Here's how the part is built. I have some questions about the finished solid (model axes, mm). Give positions to 0.01 mm unless a question says otherwise; leave off trailing zeros. Write each loop counter-clockwise with the first axis right and the second up, starting at its lowest first coordinate (ties: lowest second). Pieces come first, ordered by that corner, then holes. Notation, with made-up numbers: (-11, -6.75) - (11, -6.75) arc R26 cw to (11, 15.25) - close; hole circle Ø6 at (-28, 29.5). An arc over 180 degrees is marked (long way). One line per item, written item: value. Start each with the question number.
1) Imagine slicing it at D-D on y = 3.95. Write out the boundary of the cut face in (x, z).
2) Imagine slicing it at B-B on z = -89.34. Write out the boundary of the cut face in (x, y).
3) Please list where these lines run through material, in increasing order: L1, parallel to X at y = 1.5, z = -63; L2, parallel to X at y = 3.5, z = -129.34; L3, parallel to X at y = 1.45, z = -105. Write a range as [from, to].
4) Imagine slicing it at A-A on x = -180. Write out the boundary of the cut face in (y, z), plus the area to 3 significant figures.
5) I'm going to push a flat-ended pin straight in: P1, Ø1.8, axis at y = 2, z = -95, coming from the +X side. Where does the tip first touch, or does it pass through?
6) Imagine slicing it at C-C on z = -65. Write out the boundary of the cut face in (x, y), plus the area to 3 significant figures.
Autodesk Inventor part; units mm, degrees
ref_plane "YZ Plane" through (0, 0, 0) normal (1, 0, 0) x (0, 1, 0)
ref_plane "XZ Plane" through (0, 0, 0) normal (0, 1, 0) x (-1, 0, 0)
ref_plane "XY Plane" through (0, 0, 0) normal (0, 0, 1) x (1, 0, 0)
sketch "Sketch1" plane through (0, 0, 0) normal (0, 1, 0) x (-1, 0, 0)
  line L0 (232.1908, -176.5808) -> (232.1908, -3.7592)
  arc A0 (232.1908, -3.7592) -> (227.4316, 1) centre (227.4316, -3.7592) ccw
  line L1 (227.4316, 1) -> (0, 1)
  arc A1 (0, 1) -> (-4.7592, -3.7592) centre (0, -3.7592) ccw
  arc A2 (-4.7592, -176.5808) -> (0, -181.34) centre (0, -176.5808) ccw
  arc A3 (227.4316, -181.34) -> (232.1908, -176.5808) centre (227.4316, -176.5808) ccw
  circle A4 centre (130, -129.34) radius 2.25
  circle A5 centre (130, -89.34) radius 2.25
  circle A6 centre (90, -129.34) radius 2.25
  circle A7 centre (90, -89.34) radius 2.25
  circle A8 centre (180, -110) radius 3
  circle A9 centre (55, -110) radius 3
  circle A10 centre (90, -45) radius 3
  circle A11 centre (190, -45) radius 3
  circle A12 centre (190, -65) radius 3
  circle A13 centre (90, -65) radius 3
  circle A14 centre (140, -45) radius 3
  circle A15 centre (40, -45) radius 3
  circle A16 centre (140, -65) radius 3
  circle A17 centre (40, -65) radius 3
  line L2 (230.1908, -176.5808) -> (230.1908, -3.7592)
  arc A18 (230.1908, -3.7592) -> (227.4316, -1) centre (227.4316, -3.7592) ccw
  line L3 (227.4316, -1) -> (0, -1)
  arc A19 (0, -1) -> (-2.7592, -3.7592) centre (0, -3.7592) ccw
  arc A20 (-2.7592, -176.5808) -> (0, -179.34) centre (0, -176.5808) ccw
  arc A21 (227.4316, -179.34) -> (230.1908, -176.5808) centre (227.4316, -176.5808) ccw
  line L4 (-4.7592, -3.7592) -> (-4.7592, -176.5808)
  line L5 (-2.7592, -3.7592) -> (-2.7592, -176.5808)
  line L6 (0, -179.34) -> (227.4316, -179.34)
  line L7 (227.4316, -181.34) -> (0, -181.34)
  line L8 (0, 0) -> (0, -15)
  line L9 (0, 0) -> (15, 0) construction
  line L10 (0, 0) -> (15, 0)
  line L11 (0, 0) -> (15, 0) construction
  point P0 (230.1908, -3.7592)
  point P1 (0, -1)
  dimension "d0" = 2
  dimension "d1" = 2
  dimension "d2" = 2
  dimension "d3" = 2
  dimension "d5" = 2
  dimension "d7" = 2
  dimension "d8" = 227.4316
  dimension "d9" = 172.8216
  dimension "d10" = 4.7592
  dimension "d45" = 15
  dimension "d46" = 90
  dimension "d47" = 15
  dimension "d48" = 0
  dimension "d49" = 55
  dimension "d50" = 110
  dimension "d51" = 125
  dimension "d52" = 110
  dimension "d54" = 6
  dimension "d55" = 6
  dimension "d56" = 4.5
  dimension "d57" = 6
  dimension "d58" = 6
  dimension "d59" = 6
  dimension "d60" = 6
  dimension "d61" = 6
  dimension "d62" = 6
  dimension "d63" = 6
  dimension "d64" = 6
  dimension "d65" = 4.5
  dimension "d66" = 4.5
  dimension "d67" = 4.5
  dimension "d68" = 172.8216
  dimension "d69" = 2.7592
  dimension "d70" = 172.8216
  dimension "d71" = 2
  dimension "d72" = 1
  dimension "d73" = 230.1908
  dimension "d74" = 179.34
  dimension "d75" = 2
  dimension "d76" = 50
  dimension "d77" = 40
  dimension "d78" = 40
  dimension "d79" = 100.1908
extrude "Extrusion1" add sketch "Sketch1" along normal blind 6 contours A21 L6 A20 L5 A19 L3 A18 L2
sketch "Sketch2" plane through (0, 6, 0) normal (0, 1, 0) x (1, 0, 0)
  line L0 (-232.1908, 176.5808) -> (-232.1908, 3.7592)
  arc A0 (-232.1908, 3.7592) -> (-227.4316, -1) centre (-227.4316, 3.7592) ccw
  line L1 (-227.4316, -1) -> (0, -1)
  arc A1 (0, -1) -> (4.7592, 3.7592) centre (0, 3.7592) ccw
  arc A2 (4.7592, 176.5808) -> (0, 181.34) centre (0, 176.5808) ccw
  arc A3 (-227.4316, 181.34) -> (-232.1908, 176.5808) centre (-227.4316, 176.5808) ccw
  circle A4 centre (-130, 135) radius 2
  circle A5 centre (-130, 95) radius 2
  circle A6 centre (-90, 135) radius 2
  circle A7 centre (-90, 95) radius 2
  circle A8 centre (-160.0797, 100) radius 2.75
  circle A9 centre (-60.0797, 100) radius 2.75
  circle A10 centre (-90, 45) radius 2.5
  circle A11 centre (-190, 45) radius 2.5
  circle A12 centre (-190, 65) radius 2.5
  circle A13 centre (-90, 65) radius 2.5
  circle A14 centre (-140, 45) radius 2.5
  circle A15 centre (-40, 45) radius 2.5
  circle A16 centre (-140, 65) radius 2.5
  circle A17 centre (-40, 65) radius 2.5
  line L2 (-230.1908, 176.5808) -> (-230.1908, 3.7592)
  arc A18 (-230.1908, 3.7592) -> (-227.4316, 1) centre (-227.4316, 3.7592) ccw
  line L3 (-227.4316, 1) -> (0, 1)
  arc A19 (0, 1) -> (2.7592, 3.7592) centre (0, 3.7592) ccw
  arc A20 (2.7592, 176.5808) -> (0, 179.34) centre (0, 176.5808) ccw
  arc A21 (-227.4316, 179.34) -> (-230.1908, 176.5808) centre (-227.4316, 176.5808) ccw
  line L4 (4.7592, 3.7592) -> (4.7592, 176.5808)
  line L5 (2.7592, 3.7592) -> (2.7592, 176.5808)
  line L6 (0, 179.34) -> (-227.4316, 179.34)
  line L7 (-227.4316, 181.34) -> (0, 181.34)
  line L8 (0, 179.34) -> (-227.4316, 179.34)
  line L9 (-113.7158, 179.34) -> (-113.7158, 1)
  line L10 (-227.4316, 1) -> (0, 1)
  line L11 (-118.7158, 120.17) -> (-108.7158, 120.17)
  line L12 (-108.7158, 120.17) -> (-108.7158, 60.17)
  line L13 (-108.7158, 60.17) -> (-118.7158, 60.17)
  line L14 (-118.7158, 60.17) -> (-118.7158, 120.17)
  line L15 (-118.7158, 120.17) -> (-108.7158, 60.17) construction
  line L16 (-108.7158, 120.17) -> (-118.7158, 60.17) construction
  line L17 (-113.7158, 179.34) -> (-113.7158, 159.34)
  line L18 (2.7592, 139.34) -> (-230.1908, 139.34)
  line L19 (-230.1908, 139.34) -> (-230.1908, 179.34)
  line L20 (-230.1908, 179.34) -> (2.7592, 179.34)
  line L21 (2.7592, 179.34) -> (2.7592, 139.34)
  line L22 (2.7592, 139.34) -> (-230.1908, 179.34) construction
  line L23 (-230.1908, 139.34) -> (2.7592, 179.34) construction
  line L24 (-113.7158, 1) -> (-113.7158, 16)
  line L25 (-230.1908, 31) -> (2.7592, 31)
  line L26 (2.7592, 31) -> (2.7592, 1)
  line L27 (2.7592, 1) -> (-230.1908, 1)
  line L28 (-230.1908, 1) -> (-230.1908, 31)
  line L29 (-230.1908, 31) -> (2.7592, 1) construction
  line L30 (2.7592, 31) -> (-230.1908, 1) construction
  line L31 (-227.4316, 1) -> (0, 1)
  line L32 (-230.1908, 179.34) -> (-200.1908, 179.34)
  line L33 (-200.1908, 179.34) -> (-200.1908, 1)
  line L34 (-200.1908, 1) -> (-230.1908, 1)
  line L35 (-230.1908, 1) -> (-230.1908, 179.34)
  line L36 (2.7592, 1) -> (-27.2408, 1)
  line L37 (-27.2408, 1) -> (-27.2408, 179.34)
  line L38 (-27.2408, 179.34) -> (2.7592, 179.34)
  line L39 (2.7592, 179.34) -> (2.7592, 1)
  line L40 (-200.1908, 139.34) -> (-113.7158, 139.34)
  point P0 (230.1908, -176.5808)
  point P1 (230.1908, -3.7592)
  point P2 (227.4316, -1)
  point P3 (0, -1)
  point P4 (0, 0)
  point P5 (230.1908, -176.5808)
  point P6 (230.1908, -3.7592)
  point P7 (227.4316, -1)
  point P8 (0, -1)
  point P9 (-113.7158, 90.17)
  point P10 (-113.7158, 120.17)
  point P11 (-113.7158, 60.17)
  point P12 (-113.7158, 1)
  point P13 (0, 1)
  point P14 (-113.7158, 139.34)
  point P15 (-113.7158, 31)
  point P16 (-200.1908, 31)
  point P17 (-230.1908, 3.7592)
  point P18 (-227.4316, 1)
  dimension "d22" = 2
  dimension "d23" = 2
  dimension "d24" = 2
  dimension "d25" = 2
  dimension "d26" = 2
  dimension "d27" = 2
  dimension "d28" = 227.4316
  dimension "d29" = 172.8216
  dimension "d30" = 4.7592
  dimension "d31" = 10
  dimension "d32" = 60
  dimension "d37" = 20
  dimension "d38" = 40
  dimension "d39" = 15
  dimension "d40" = 30
  dimension "d41" = 30
  dimension "d42" = 30
extrude "Extrusion3" cut sketch "Sketch2" against normal through all contours A6 | A7 | A9 | A10 | A13 | A15 | A17 | A21 L6 L33 L18 L2 | L18 L33 L25 L2 | L25 L33 L3 A18 L2 | L33 L6 L9 L18 | L25 L9 L3 L33 | L18 L37 L25 L9 L13 L12 L11 | L9 L6 L37 L18 | L25 L37 L3 L9 | L11 L12 L13 L9 | L9 L13 L14 L11 | L37 L6 A20 L5 L18 | L18 L5 L25 L37 | L25 L5 A19 L3 L37
fillet "Fillet3" radius 2 6 edges at (-113.7158, 3, -31) (-200.1908, 3, -31) (-113.7158, 3, -139.34) (-118.7158, 3, -120.17) (-118.7158, 3, -60.17) (-200.1908, 3, -139.34)
equation "\"d1\" = d0"
equation "\"d2\" = d0"
equation "\"d3\" = d0"
equation "\"d5\" = d0"
equation "\"d7\" = d0"
equation "\"d23\" = d22"
equation "\"d24\" = d22"
equation "\"d25\" = d22"
equation "\"d26\" = d22"
equation "\"d27\" = d22"
properties part number "EboxBottom_1"
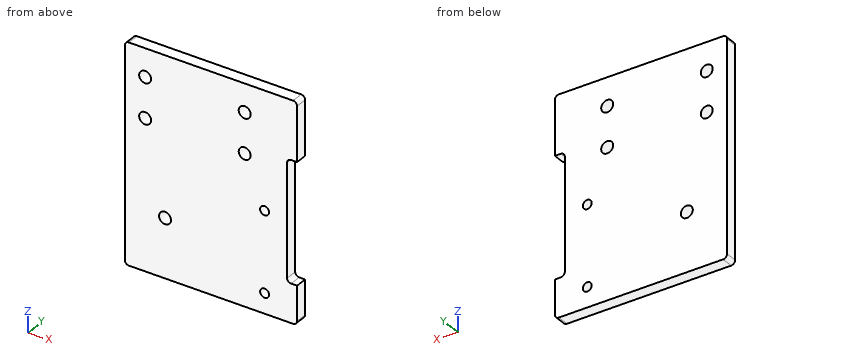
Numbers:
1. outline: (-200.19, -137.34) arc R2 ccw to (-198.19, -139.34) - (-115.72, -139.34) arc R2 ccw to (-113.72, -137.34) - (-113.72, -120.17) - (-116.72, -120.17) arc R2 cw to (-118.72, -118.17) - (-118.72, -62.17) arc R2 cw to (-116.72, -60.17) - (-113.72, -60.17) - (-113.72, -33) arc R2 ccw to (-115.72, -31) - (-198.19, -31) arc R2 ccw to (-200.19, -33) - close; hole circle Ø6 at (-190, -65); hole circle Ø6 at (-190, -45); hole circle Ø6 at (-180, -110); hole circle Ø6 at (-140, -65); hole circle Ø6 at (-140, -45); hole circle Ø4.5 at (-130, -129.34); hole circle Ø4.5 at (-130, -89.34)
2. outline: (-200.19, 0) - (-132.25, 0) - (-132.25, 6) - (-200.19, 6) - close; (-127.75, 0) - (-118.72, 0) - (-118.72, 6) - (-127.75, 6) - close
3. L1: [-200.19, -192.24], [-187.76, -142.24], [-137.76, -118.72]
3. L2: [-200.19, -132.25], [-127.75, -113.72]
3. L3: [-200.19, -118.72]
4. outline: (0, -139.34) - (6, -139.34) - (6, -113) - (0, -113) - close; (0, -107) - (6, -107) - (6, -31) - (0, -31) - close
4. area: 614 mm^2
5. P1: x = -118.72
6. outline: (-200.19, 0) - (-193, 0) - (-193, 6) - (-200.19, 6) - close; (-187, 0) - (-143, 0) - (-143, 6) - (-187, 6) - close; (-137, 0) - (-118.72, 0) - (-118.72, 6) - (-137, 6) - close
6. area: 417 mm^2
